Check sheet for the drawn part. Datum: minimum x, y, z corner. Units: mm. Coordinates: 2 decimals unless noted, no trailing zeros. Write each loop counter-clockwise with the first axis right and the second up, starting at its lowest first coordinate (ties: lowest second). Pieces come first, ordered by that corner, then holes. Notation, with made-up numbers: (34.25, -14.5) -> (92.25, -14.5) arc R17 cw to (92.25, 16.5) -> close; hole circle Ø11 at (45.25, 47). An arc over 180 degrees is marked (long way). Answer in a Markdown table with one row per item.
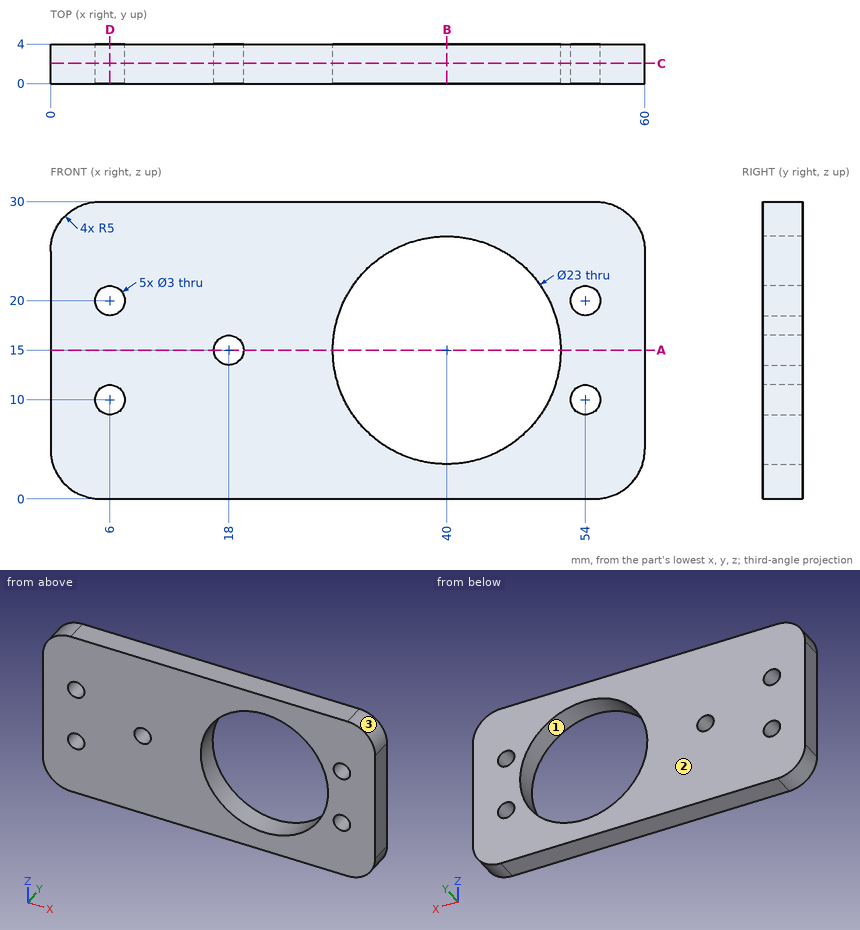
1. Release check for a two-part mould opening along X. For the marked faces 1, 2 and 3 record: released by +X, released by -X, zero draft, split by the parting line, or undercut.
Findings below:
| item | result |
|---|---|
| face 1 | undercut |
| face 2 | zero draft |
| face 3 | released by +X |
2. Material ranges on probe 1 along X at (y, z) = (2.3, 15); probe 2 along X at (y, z) = (3, 20); probe 3 along X at (y, z) = (1.35, 19.75), recorded low to high. Write a range as from..to.
Findings below:
| item | result |
|---|---|
| probe 1 | x = 0..16.5, 19.5..28.5, 51.5..60 |
| probe 2 | x = 0..4.5, 7.5..29.64, 50.36..52.5, 55.5..60 |
| probe 3 | x = 0..4.52, 7.48..29.53, 50.47..52.52, 55.48..60 |
3. Go/stop test with a flat-tipped pin: pin 1 (1.5 mm diameter, centred on y = 3.5, z = 3.5, fed in from -X). Record where the tip stops, or that it passes through.
Findings below:
| item | result |
|---|---|
| pin 1 | stops at x = 0.06 |
4. Sectioned sample at A-A, the plane z = 15. Record the cut outline in (x, y), and give its area (3 significant figures).
Findings below:
| item | result |
|---|---|
| outline | (0, 0) -> (16.5, 0) -> (16.5, 4) -> (0, 4) -> close; (19.5, 0) -> (28.5, 0) -> (28.5, 4) -> (19.5, 4) -> close; (51.5, 0) -> (60, 0) -> (60, 4) -> (51.5, 4) -> close |
| area | 136 mm² |
5. Sectioned sample at D-D, the plane x = 6. Record the cut outline in (y, z), and give its area (3 significant figures).
Findings below:
| item | result |
|---|---|
| outline | (0, 0) -> (4, 0) -> (4, 8.5) -> (0, 8.5) -> close; (0, 11.5) -> (4, 11.5) -> (4, 18.5) -> (0, 18.5) -> close; (0, 21.5) -> (4, 21.5) -> (4, 30) -> (0, 30) -> close |
| area | 96.0 mm² |
6. Sectioned sample at B-B, the plane x = 40. Record the cut outline in (y, z).
Findings below:
| item | result |
|---|---|
| outline | (0, 0) -> (4, 0) -> (4, 3.5) -> (0, 3.5) -> close; (0, 26.5) -> (4, 26.5) -> (4, 30) -> (0, 30) -> close |
7. Sectioned sample at C-C, the plane y = 2.05. Record the cut outline in (x, z), and give its area (3 significant figures).
Findings below:
| item | result |
|---|---|
| outline | (0, 5) arc R5 ccw to (5, 0) -> (55, 0) arc R5 ccw to (60, 5) -> (60, 25) arc R5 ccw to (55, 30) -> (5, 30) arc R5 ccw to (0, 25) -> close; hole circle Ø3 at (6, 10); hole circle Ø3 at (6, 20); hole circle Ø3 at (18, 15); hole circle Ø23 at (40, 15); hole circle Ø3 at (54, 10); hole circle Ø3 at (54, 20) |
| area | 1,330 mm² |
